Autodesk Inventor part; units mm, degrees
ref_plane "YZ Plane" through (0, 0, 0) normal (1, 0, 0) x (0, 1, 0)
ref_plane "XZ Plane" through (0, 0, 0) normal (0, 1, 0) x (-1, 0, 0)
ref_plane "XY Plane" through (0, 0, 0) normal (0, 0, 1) x (1, 0, 0)
sketch "Sketch1" plane through (0, 0, 0) normal (0, 0, 1) x (1, 0, 0)
  line L0 (-73.5, -17) -> (73.5, -17)
  line L1 (73.5, -17) -> (73.5, 17)
  line L2 (73.5, 17) -> (-73.5, 17)
  line L3 (-73.5, 17) -> (-73.5, -17)
  line L4 (-73.5, -17) -> (73.5, 17) construction
  line L5 (73.5, -17) -> (-73.5, 17) construction
  point P0 (0, 0)
  dimension "d0" = 147
  dimension "d1" = 34
extrude "Extrusion1" add sketch "Sketch1" along normal blind 6
sketch "Sketch2" plane through (0, 0, 6) normal (0, 0, 1) x (1, 0, 0)
  line L0 (-37, -10) -> (37, -10)
  line L1 (37, -10) -> (37, 10)
  line L2 (37, 10) -> (-37, 10)
  line L3 (-37, 10) -> (-37, -10)
  line L4 (-37, -10) -> (37, 10) construction
  line L5 (37, -10) -> (-37, 10) construction
  point P0 (0, 0)
  dimension "d4" = 74
  dimension "d5" = 20
extrude "Extrusion2" cut sketch "Sketch2" against normal blind 6
sketch "Sketch3" plane through (0, 0, 6) normal (0, 0, 1) x (1, 0, 0)
  circle A0 centre (0, 9) radius 2.5
  circle A1 centre (0, -9) radius 2.5
  point P0 (0, 0)
  dimension "d8" = 5
  dimension "d10" = 9
  dimension "d11" = 5
  dimension "d12" = 9
extrude "Extrusion3" cut sketch "Sketch3" against normal blind 6
sketch "Sketch4" plane through (0, 0, 6) normal (0, 0, 1) x (1, 0, 0)
  line L0 (73.5, 17) -> (-73.5, 17)
  circle A0 centre (-50, 19) radius 3
  line L1 (-56, 13) -> (-44, 13)
  line L2 (-44, 13) -> (-44, 25)
  line L3 (-44, 25) -> (-56, 25)
  line L4 (-56, 25) -> (-56, 13)
  line L5 (-56, 13) -> (-44, 25) construction
  line L6 (-44, 13) -> (-56, 25) construction
  point P0 (0, 0)
  dimension "d15" = 6
  dimension "d16" = 12
  dimension "d17" = 12
  dimension "d18" = 50
  dimension "d19" = 2
extrude "Extrusion4" add sketch "Sketch4" against normal blind 6 contours L2 L1 L4 L0 A0 | L0 A0 L4 L3 L2
sketch "Sketch5" plane through (0, 0, 6) normal (0, 0, 1) x (1, 0, 0)
  line L0 (-73.5, 17) -> (-73.5, -17)
  line L1 (-37, -10) -> (-37, 10)
  line L2 (-73.5, 5) -> (-64.5, 5)
  line L3 (-64.5, 5) -> (-64.5, -5)
  line L4 (-64.5, -5) -> (-73.5, -5)
  line L5 (-73.5, -5) -> (-73.5, 5)
  point P0 (0, 0)
  point P1 (-73.5, 0)
  point P2 (-37, 0)
  dimension "d22" = 9
  dimension "d23" = 10
extrude "Extrusion5" cut sketch "Sketch5" against normal blind 6
sketch "Sketch6" plane through (0, 0, 6) normal (0, 0, 1) x (1, 0, 0)
  line L0 (-73.5, -17) -> (-49.5, -17)
  line L1 (-49.5, -17) -> (-49.5, -10)
  line L2 (-49.5, -10) -> (-73.5, -10)
  line L3 (-73.5, -10) -> (-73.5, -17)
  point P0 (0, 0)
  dimension "d26" = 24
  dimension "d28" = 7
extrude "Extrusion6" cut sketch "Sketch6" against normal blind 6
sketch "Sketch7" plane through (0, 0, 6) normal (0, 0, 1) x (1, 0, 0)
  line L0 (-37, -10) -> (-37, 10)
  circle A0 centre (-44.1, 0) radius 1.125
  point P0 (0, 0)
  point P1 (-37, 0)
  dimension "d31" = 2.25
  dimension "d32" = 44.1
extrude "Extrusion7" cut sketch "Sketch7" against normal blind 6
mirror "Mirror1" about plane through (0, 0, 0) normal (1, 0, 0) of "Extrusion4", "Extrusion5", "Extrusion6", "Extrusion7"
chamfer "Chamfer3" distance 5 angle 45 2 edges at (-37, 10, 3) (37, 10, 3)
chamfer "Chamfer4" distance 2 angle 45 4 edges at (-37, -10, 3) (-49.5, -10, 3) (37, -10, 3) (49.5, -10, 3)
fillet "Fillet2" radius 3 12 edges at (-73.5, 17, 3) (-56, 17, 3) (-56, 25, 3) (-44, 25, 3) (-44, 17, 3) (-49.5, -17, 3) (49.5, -17, 3) (73.5, 17, 3) (56, 17, 3) (56, 25, 3) (44, 25, 3) (44, 17, 3)
sketch "Sketch8" plane through (0, 0, 6) normal (0, 0, 1) x (1, 0, 0)
  circle A0 centre (50, 19) radius 3
  circle A1 centre (-50, 19) radius 3
  arc A2 (-47.7639, 17) -> (-52.2361, 17) centre (-50, 19) ccw
  arc A3 (52.2361, 17) -> (47.7639, 17) centre (50, 19) ccw
  point P0 (0, 0)
extrude "Extrusion8" cut sketch "Sketch8" against normal through all
properties part number "camera_mount_v1"
Build history of the part. All positions in model axes, mm. A direction names the side the tool comes from. Give positions to 0.01 mm unless a question says otherwise; leave off trailing zeros. Loops run counter-clockwise (first coordinate to the right, second up) from the corner with the lowest first, then second, coordinate; pieces in that order, holes last.
1) Band-saw the part on B-B on x = 9.5. List the corners of the cut face in (y, z).
Values follow:
outline: (-17, 0) - (-10, 0) - (-10, 6) - (-17, 6) - close; (10, 0) - (17, 0) - (17, 6) - (10, 6) - close
2) Two-plate mould, pull along Y, no slides. Class faces 1 (the face through (-1, -17, 3)), 2 (the face through (-43.14, 17.9, 3.04)), 3 (the face through (0, -11.5, 3)): released by +Y, released by -Y, zero draft, split by the parting line, or undercut.
Values follow:
face 1: released by -Y
face 2: released by +Y
face 3: undercut
3) 3-axis set-ups, long thin cutter, end or side, ignore diameter. For faces 4 (the face through (64.5, 0, 3)), 5 (the face through (-44.9, 24.14, 2.96)), 6 (the face through (-69, 5, 3)), 7 (the face through (-17, 10, 3)): which of +Z, -Z, +X, -X, +Y, -Y reach the whole face in a straight line?
Values follow:
face 4: +Z, -Z, +X
face 5: +Z, -Z, +Y
face 6: +Z, -Z, -X
face 7: +Z, -Z
4) Drop flat-ended pins along their axis: P1, Ø1, axis at y = 1, z = 3, coming from the -X side; P2, Ø1.5, axis at x = 5.5, z = 2, coming from the +Y side; P3, Ø2, axis at y = 21, z = 3, coming from the -X side. Give the stop position or say it passes through.
Values follow:
P1: stops at x = -64.5
P2: stops at y = 17
P3: stops at x = -56
5) Band-saw the part on D-D on z = 4.8. State how many separate pieces and enclosed holes the cut face has, then the cut area to 3 significant figures.
Values follow:
separate pieces: 1
enclosed holes: 5
area: 3,140 mm2
6) Band-saw the part on A-A on y = 7. List the corners of the cut face in (x, z).
Values follow:
outline: (-73.5, 0) - (-35, 0) - (-35, 6) - (-73.5, 6) - close; (35, 0) - (73.5, 0) - (73.5, 6) - (35, 6) - close
7) Band-saw the part on C-C on x = -39. List the corners of the cut face in (y, z).
Values follow:
outline: (-17, 0) - (17, 0) - (17, 6) - (-17, 6) - close
8) Probe line 1 along Y through (x, z) = (-50, 4.5); line 2 along X through (y, z) = (-7, 4.5); line 3 along Y through (x, z) = (13.5, 2.55). List the from-to ranges inside material, lowest first.
Values follow:
line 1: y = -11.5 to 16, 22 to 25
line 2: x = -73.5 to -37, 37 to 73.5
line 3: y = -17 to -10, 10 to 17
